Autodesk Inventor part; units mm, degrees
ref_plane "YZ Plane" through (0, 0, 0) normal (1, 0, 0) x (0, 1, 0)
ref_plane "XZ Plane" through (0, 0, 0) normal (0, 1, 0) x (-1, 0, 0)
ref_plane "XY Plane" through (0, 0, 0) normal (0, 0, 1) x (1, 0, 0)
sketch "Sketch1" plane through (0, 0, 0) normal (0, 1, 0) x (-1, 0, 0)
  line L0 (0, 0) -> (1219.2, 0)
  line L1 (1219.2, 0) -> (1422.4, 351.9527)
  line L2 (1422.4, 351.9527) -> (812.8, 1407.8109)
  line L3 (812.8, 1407.8109) -> (406.4, 1407.8109)
  line L4 (406.4, 1407.8109) -> (-203.2, 351.9527)
  line L5 (-203.2, 351.9527) -> (0, 0)
  dimension "d7" = 1219.2
  dimension "d8" = 406.4
  dimension "d9" = 120
  dimension "d10" = 1219.2
  dimension "d11" = 120
  dimension "d12" = 406.4
  dimension "d13" = 1219.2
  dimension "d14" = 120
extrude "Plate1" add sketch "Sketch1" along normal blind 3.048
equation "\"BendRadius\" = Thickness"
equation "\"BendReliefWidth\" = Thickness"
equation "\"BendReliefDepth\" = 0.5 * Thickness"
equation "\"CornerReliefSize\" = 4 * Thickness"
equation "\"MinimumRemnant\" = 2 * Thickness"
equation "\"TransitionRadius\" = BendRadius"
equation "\"JacobiRadiusSize\" = BendRadius"
equation "\"GapSize\" = Thickness"
equation "\"d2\" = BendRadius"
properties part number "Ground" material "Carpet"
Geometry check sheet. Reference: the model listing, model coordinates, mm. Give positions to 0.01 mm unless a question says otherwise; leave off trailing zeros. Write each loop counter-clockwise with the first axis right and the second up, starting at its lowest first coordinate (ties: lowest second). Pieces come first, ordered by that corner, then holes. Notation, with made-up numbers: (62, 81) - (119, 81) arc R28 cw to (119, 102) - close; hole circle Ø6 at (88.25, 80). An arc over 180 degrees is marked (long way). Use a Markdown table: item, result.
Q1. Section check C-C, the plane x = -1270. Enter the section's corners in (y, z).
Computed:
| item | result |
|---|---|
| outline | (0, 87.99) - (3.05, 87.99) - (3.05, 615.92) - (0, 615.92) - close |
Q2. Section check B-B, the plane z = 486.5. Enter the section's corners in (x, y), then the cut area to 3 significant figures.
Computed:
| item | result |
|---|---|
| outline | (-1344.72, 0) - (125.52, 0) - (125.52, 3.05) - (-1344.72, 3.05) - close |
| area | 4,480 mm² |
Q3. Thickness scan on L1, parallel to Z at x = -25, y = 2.15; L2, parallel to Z at x = -269, y = 1.55; L3, parallel to X at y = 1.5, z = 763. Record the ranges inside material, lowest first. Write a range as [from, to].
Computed:
| item | result |
|---|---|
| L1 | z = [0, 747.21] |
| L2 | z = [0, 1169.83] |
| L3 | x = [-1185.08, -34.12] |
Q4. Go/stop test with flat-tipped pins: P1, Ø1.5, axis at y = 2, z = 539.5, coming from the -X side; P2, Ø1.5, axis at y = 2, z = 387, coming from the -X side. Record where each tip stops, or that it passes through.
Computed:
| item | result |
|---|---|
| P1 | stops at x = -1314.55 |
| P2 | stops at x = -1402.6 |
Q5. Section check A-A, the plane y = 1.85. Enter the section's corners in (x, z), then the cut area to 3 significant figures.
Computed:
| item | result |
|---|---|
| outline | (-1422.4, 351.95) - (-1219.2, 0) - (0, 0) - (203.2, 351.95) - (-406.4, 1407.81) - (-812.8, 1407.81) - close |
| area | 1,570,000 mm² |
